from build123d import *

# Parameters (mm, degrees)
SKETCH1_R           = 13
SKETCH1_R_2         = 8
BOSS_EXTRUDE1_DEPTH = 10


with BuildPart() as part:
    # Sketch1 → Boss-Extrude1 (new body)
    # profile 1 of 5: a face of its own
    with BuildSketch(Plane(origin=(0, 0, 0), x_dir=(1, 0, 0), z_dir=(0, 1, 0))):
        with Locations((5, -16)):
            Circle(SKETCH1_R)
        with Locations(Location((5, -16, 0), (0, 0, 270))):
            Circle(SKETCH1_R_2, mode=Mode.SUBTRACT)
    # profile 2 of 5: a face of its own
    with BuildSketch(Plane(origin=(0, 0, 0), x_dir=(1, 0, 0), z_dir=(0, 1, 0))):
        with BuildLine():
            Line((10, -3), (5, -3))
            ThreePointArc((5, -3), (9.666728031, -3.866507119), (13.711340206, -6.350515464))
            Line((13.711340206, -6.350515464), (10, -3))
        make_face()
    # profile 3 of 5: a face of its own
    with BuildSketch(Plane(origin=(0, 0, 0), x_dir=(1, 0, 0), z_dir=(0, 1, 0))):
        Polygon((7.5, 5), (5, 5), (5, -3), (10, -3), (10, 0), (6.5, 0), align=None)
    # profile 4 of 5: a face of its own
    with BuildSketch(Plane(origin=(0, 0, 0), x_dir=(1, 0, 0), z_dir=(0, 1, 0))):
        Polygon((2.5, 5), (3.5, 0), (0, 0), (0, -3), (5, -3), (5, 5), align=None)
    # profile 5 of 5: a face of its own
    with BuildSketch(Plane(origin=(0, 0, 0), x_dir=(1, 0, 0), z_dir=(0, 1, 0))):
        with BuildLine():
            Line((5, -3), (0, -3))
            Line((0, -3), (-3.711340206, -6.350515464))
            ThreePointArc((-3.711340206, -6.350515464), (0.333271969, -3.866507119), (5, -3))
        make_face()
    extrude(amount=BOSS_EXTRUDE1_DEPTH)


solid = part.part
Could you check a few things on this model? Use its own coordinates, in mm. A direction names the side the tool comes from. Give positions to 0.01 mm unless a question says otherwise; leave off trailing zeros. Order: outer loops, then holes, each group sorted by start corner. A loop starts at its lowest first (then second) coordinate and runs counter-clockwise, first axis right, second up.
1. Suppose I cut it at C-C (y = 2.5). Write out the boundary of the cut face in (x, z), plus the area to 3 significant figures.
Answers below:
outline: (-3.71, 6.35) - (0, 3) - (0, 0) - (3.5, 0) - (2.5, -5) - (7.5, -5) - (6.5, 0) - (10, 0) - (10, 3) - (13.71, 6.35) arc R13 ccw (long way) to start; hole circle Ø16 at (5, 16)
area: 386 mm2
2. Suppose I cut it at A-A (z = 16). Write out the boundary of the cut face in (x, y), plus the area to 3 significant figures.
Answers below:
outline: (-8, 0) - (-3, 0) - (-3, 10) - (-8, 10) - close; (13, 0) - (18, 0) - (18, 10) - (13, 10) - close
area: 100 mm2
3. For pin 1 (2 mm diameter, centred on y = 1.5, z = 13.5, fed in from -X); pin 2 (1.8 mm diameter, centred on x = 1, y = 3.5, fed in from -Z); pin 3 (1.5 mm diameter, centred on y = 5.5, z = 2, fed in from +X), each with a flat end and sliding along its axis, tell me the tip position at first contact or that it passes through.
Answers below:
pin 1: stops at x = -7.91
pin 2: stops at z = 0
pin 3: stops at x = 10
4. Thinking about a two-plate mould opening in Z: for faces 1 (the flat face through (10, 5, 2)), 2 (the flat face through (7, 4.9, -2.5)), 3 (the cylindrical face through (5, 5, 29)), which applies, +Z half, -Z half, draft (parallel to the pull), parting line (faces both ways), or undercut?
Answers below:
face 1: draft
face 2: undercut
face 3: parting line
5. Suppose I cut it at D-D (z = 0.5). Write out the boundary of the cut face in (x, y), plus the area to 3 significant figures.
Answers below:
outline: (0, 0) - (10, 0) - (10, 10) - (0, 10) - close
area: 100 mm2
6. Suppose I cut it at B-B (x = 5). Write out the boundary of the cut face in (y, z), plus the area to 3 significant figures.
Answers below:
outline: (0, -5) - (10, -5) - (10, 8) - (0, 8) - close; (0, 24) - (10, 24) - (10, 29) - (0, 29) - close
area: 180 mm2
7. Which directions (+Z, -Z, +X, -X, +Y, -Y) give clear straight access to the entire face, cutting with the end or side of a thin tool? Please do faces 4 (the flat face through (8, 5, 0)), 5 (the flat face through (0, 5, 1)), 6 (the flat face through (3, 4.9, -2.5)), 7 (the flat face through (8, 0, 8)).
Answers below:
face 4: +X, +Y, -Y
face 5: -Z, -X, +Y, -Y
face 6: -X, +Y, -Y
face 7: +Z, -Z, +X, -X, -Y
8. I need wall thicknesses on L1, parallel to X at y = 7.75, z = 16; L2, parallel to X at y = 4.75, z = 18; L3, parallel to Z at x = -5.25, y = 1.75. Which ranges of each line are inside material? Lowest first, please.
Answers below:
L1: x = -8 to -3, 13 to 18
L2: x = -7.85 to -2.75, 12.75 to 17.85
L3: z = 8 to 24
